Input: dimensioned drawing with shaded views. Units: mm. Origin: part minimum x, y, z. A direction names the side the tool comes from. Give positions to 0.01 mm unless a question says otherwise; leave off trailing zeros. Loops run counter-clockwise (first coordinate to the right, second up) from the corner with the lowest first, then second, coordinate; pieces in that order, holes last.
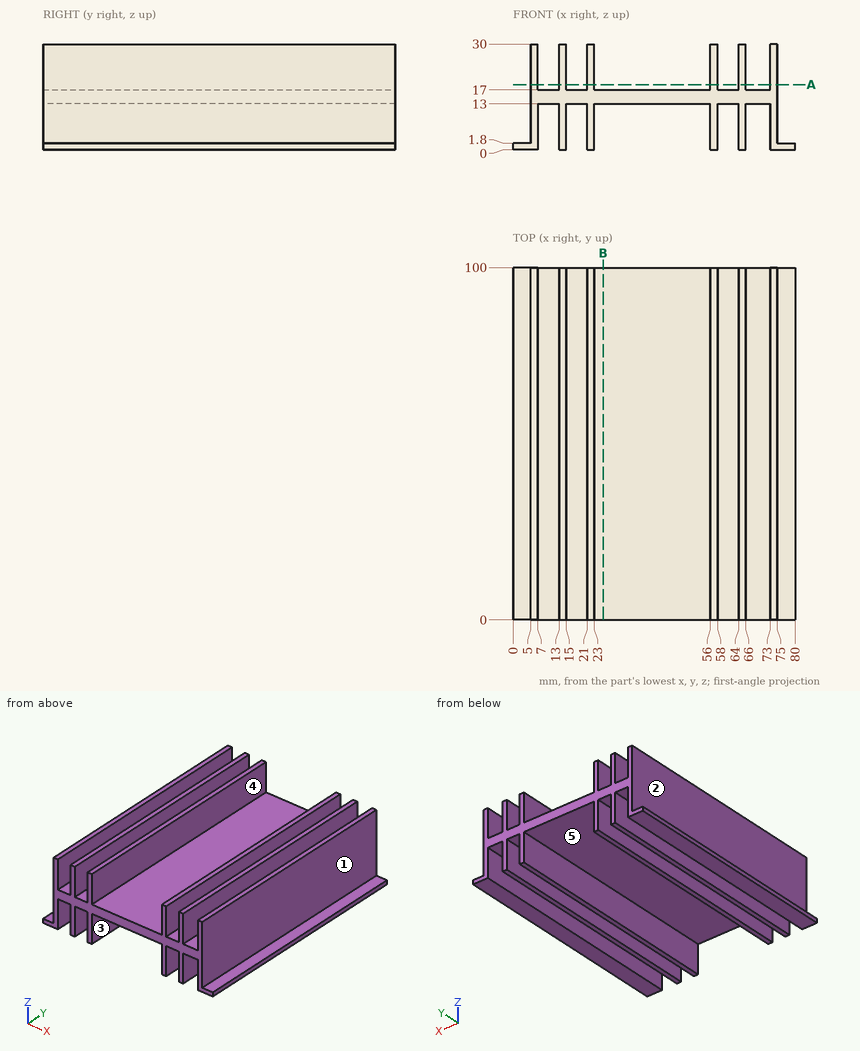
Item 1: Section query B-B on x = 25.5. Return loops of the section in (y, z).
Values follow:
outline: (0, 13) - (100, 13) - (100, 17) - (0, 17) - close
Item 2: Ray query, probe 1 along X at (y, z) = (33.5, 20.25); probe 2 along Z at (x, y) = (16, 57.5); probe 3 along X at (y, z) = (89, 15). Return the intervals inside material, ascending.
Values follow:
probe 1: x = 5 to 7, 13 to 15, 21 to 23, 56 to 58, 64 to 66, 73 to 75
probe 2: z = 13 to 17
probe 3: x = 5 to 75
Item 3: Section query A-A on z = 18.5. Return loops of the section in (x, y), plus the area to 3 significant figures.
Values follow:
outline: (5, 0) - (7, 0) - (7, 100) - (5, 100) - close; (13, 0) - (15, 0) - (15, 100) - (13, 100) - close; (21, 0) - (23, 0) - (23, 100) - (21, 100) - close; (56, 0) - (58, 0) - (58, 100) - (56, 100) - close; (64, 0) - (66, 0) - (66, 100) - (64, 100) - close; (73, 0) - (75, 0) - (75, 100) - (73, 100) - close
area: 1,200 mm2
Item 4: Draft query along X for the marked faces 1, 2 and 3. Return one class per face: +X half, -X half, draft (parallel to the pull), parting line (faces both ways), or undercut.
Values follow:
face 1: +X half
face 2: -X half
face 3: undercut
Item 5: Pin query (flat end, axial travel): pin 1 (14.5 mm diameter, centred on y = 62.5, z = 22, fed in from +X); pin 2 (10.5 mm diameter, centred on y = 70.5, z = 25.5, fed in from -X); pin 3 (5.5 mm diameter, centred on x = 2, y = 31, fed in from +Z). Return the tip coordinate at first contact, or that it passes through.
Values follow:
pin 1: stops at x = 75
pin 2: stops at x = 5
pin 3: stops at z = 1.8
Item 6: Set-up query: the marked faces 4 and 5. Return all of +Z, -Z, +X, -X, +Y, -Y with unobstructed straight access to the full face (end or side cutting, diameter ignored); none if empty.
Values follow:
face 4: +Z, +Y, -Y
face 5: -Z, +Y, -Y
